Work out the finished part from the listing and answer in its coordinate system (mm). Face numbers are marked on the shaded views. A direction names the side the tool comes from. Coordinates: 2 decimals unless noted, no trailing zeros. Order: outer loops, then holes, each group sorted by start corner. A loop starts at its lowest first (then second) coordinate and runs counter-clockwise, first axis right, second up. Notation, with made-up numbers: M -2,55.5 L 28,55.5 A16 ccw 28,71.5 Z; hole C 20.5,29.5 d6. An arc over 180 degrees is marked long. Answer in a Markdown table with one row per item. Add a question column.
Item 1: The part is cut by section A-A (y = 8). Write down the section's boundary in (x, z).
Item 2: A flat-ended cylindrical pin translates along its axis: pin 1 Ø8 at (x, z) = (-12, 9.5) entering from +Y. Find the tip coordinate at first contact, or state that the pin passes through.
Item 3: Consider line 1 (X direction, y = 15.5, z = 17); line 2 (Z direction, x = -11.5, y = 36.5); line 3 (X direction, y = 27.5, z = 32). Determine where each line is inside the solid, lowest interval first. Write a range as from..to.
Item 4: The part is cut by section B-B (x = 34). Write down the section's boundary in (y, z).
Item 5: The part is cut by section D-D (z = 4). Write down the section's boundary in (x, y), then the cut area to 3 significant figures.
Item 6: The part is cut by section C-C (y = 21). Write down the section's boundary in (x, z).
Item 7: Which of the six approach directions +Z, -Z, +X, -X, +Y, -Y give full straight-line access (tool end or side, diameter ignored) to the marked faces 1 and 2?
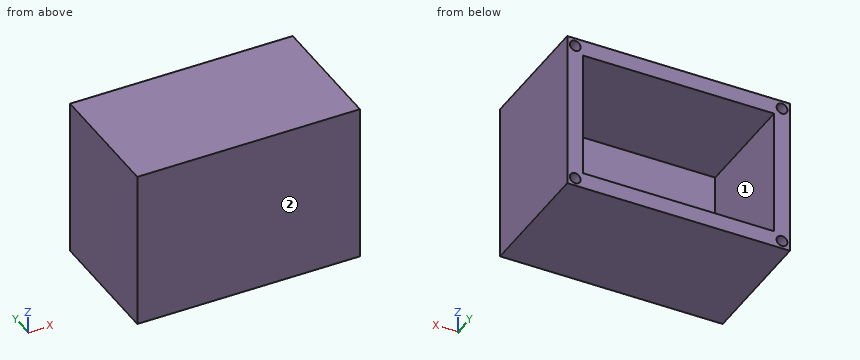
from build123d import *

# Parameters (mm, degrees)
CROQUIS1_W                       = 70
CROQUIS1_H                       = 50
SALIENTE_EXTRUIR1_DEPTH          = 40
CROQUIS2_W                       = 60
CROQUIS2_H                       = 40
CORTAR_EXTRUIR1_DEPTH            = 71.017609314
CROQUIS3_W                       = 60
CROQUIS3_H                       = 40
SALIENTE_EXTRUIR2_DEPTH          = 5
TALADRO_DE_MARGEN_PARA_M31_D     = 3.4
TALADRO_DE_MARGEN_PARA_M31_DEPTH = 20
TALADRO_DE_MARGEN_PARA_M31_TIP   = 1.021463052


with BuildPart() as part:
    # Croquis1 → Saliente-Extruir1 (new body)
    with BuildSketch(Plane(origin=(0, 0, 0), x_dir=(1, 0, 0), z_dir=(0, 1, 0))):
        with Locations((10.018270402, -10.71863581)):
            Rectangle(CROQUIS1_W, CROQUIS1_H)
    extrude(amount=SALIENTE_EXTRUIR1_DEPTH)

    # Croquis2 → Cortar-Extruir1 (cut, through all)
    with BuildSketch(Plane(origin=(0, 0, 0), x_dir=(1, 0, 0), z_dir=(0, 1, 0))):
        with Locations((10.018270402, -10.71863581)):
            Rectangle(CROQUIS2_W, CROQUIS2_H)
    extrude(amount=CORTAR_EXTRUIR1_DEPTH, mode=Mode.SUBTRACT)

    # Croquis3 → Saliente-Extruir2 (add)
    with BuildSketch(Plane(origin=(0, 0, 0), x_dir=(1, 0, 0), z_dir=(0, 1, 0))):
        with Locations((10.018270402, -10.71863581)):
            Rectangle(CROQUIS3_W, CROQUIS3_H)
    extrude(amount=SALIENTE_EXTRUIR2_DEPTH)

    # Taladro de margen para M31
    with Locations(Plane(origin=(-22.481719301, 40, -11.781363893), x_dir=(0, 0, 1), z_dir=(0, 1, 0))):
        with Locations((0, 0), (-2.33e-07, 64.999991125), (44.999999703, 64.999989703), (45.0000013, 65.000000057), (45.000001979, 1.038e-06)):
            Hole(TALADRO_DE_MARGEN_PARA_M31_D / 2, depth=TALADRO_DE_MARGEN_PARA_M31_DEPTH)
            with Locations((0, 0, -(TALADRO_DE_MARGEN_PARA_M31_DEPTH + TALADRO_DE_MARGEN_PARA_M31_TIP / 2))):  # 118° drill point
                Cone(0, TALADRO_DE_MARGEN_PARA_M31_D / 2, TALADRO_DE_MARGEN_PARA_M31_TIP, mode=Mode.SUBTRACT)


solid = part.part
Reply:
| question | item | result |
|---|---|---|
| 1 | outline | M -24.98,-14.28 L 45.02,-14.28 L 45.02,35.72 L -24.98,35.72 Z; hole M -19.98,-9.28 L 40.02,-9.28 L 40.02,30.72 L -19.98,30.72 Z |
| 2 | pin 1 | stops at y = 5 |
| 3 | line 1 | x = -24.98..-19.98, 40.02..45.02 |
| 3 | line 2 | z = -14.28..-9.28, 30.72..35.72 |
| 3 | line 3 | x = -24.98..-23.67, -21.3..41.33, 43.7..45.02 |
| 4 | outline | M 0,-14.28 L 40,-14.28 L 40,-9.28 L 5,-9.28 L 5,30.72 L 40,30.72 L 40,35.72 L 0,35.72 Z |
| 5 | outline | M -24.98,0 L 45.02,0 L 45.02,40 L 40.02,40 L 40.02,5 L -19.98,5 L -19.98,40 L -24.98,40 Z |
| 5 | area | 700 mm2 |
| 6 | outline | M -24.98,-14.28 L 45.02,-14.28 L 45.02,35.72 L -24.98,35.72 Z; hole C -22.48,-11.78 d3.4; hole C -22.48,33.22 d3.4; hole M -19.98,-9.28 L 40.02,-9.28 L 40.02,30.72 L -19.98,30.72 Z; hole C 42.52,-11.78 d3.4; hole M 42.26,34.9 A1.7 ccw 42.78,31.54 A1.7 ccw Z |
| 7 | face 1 | +Y |
| 7 | face 2 | +Z, -Z, +X, -X, -Y |
